```python
from build123d import *

# Parameters (mm, degrees)
SKETCH1_W           = 20
SKETCH1_H           = 20
BOSS_EXTRUDE1_DEPTH = 20
SKETCH2_W           = 10
SKETCH2_H           = 10
CUT_EXTRUDE1_DEPTH  = 20
CUT_EXTRUDE2_DEPTH  = 20


with BuildPart() as part:
    # Sketch1 → Boss-Extrude1 (new body)
    with BuildSketch(Plane.XY):
        with Locations((10, 10)):
            Rectangle(SKETCH1_W, SKETCH1_H)
    extrude(amount=BOSS_EXTRUDE1_DEPTH)

    # Sketch2 → Cut-Extrude1 (cut)
    with BuildSketch(Plane(origin=(0, 20, 0), x_dir=(1, 0, 0), z_dir=(0, 1, 0))):
        with Locations((5, -15)):
            Rectangle(SKETCH2_W, SKETCH2_H)
    extrude(amount=-CUT_EXTRUDE1_DEPTH, mode=Mode.SUBTRACT)

    # Sketch3 → Cut-Extrude2 (cut)
    with BuildSketch(Plane(origin=(0, 20, 0), x_dir=(1, 0, 0), z_dir=(0, 1, 0))):
        Polygon((0, 0), (10, -10), (0, -10), align=None)
    extrude(amount=-CUT_EXTRUDE2_DEPTH, mode=Mode.SUBTRACT)


solid = part.part
```
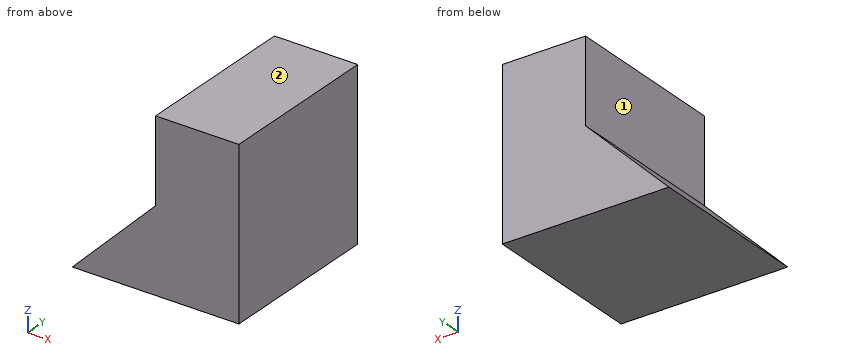
Here's how the part is built. I have some questions about the finished solid (model axes, mm). Face numbers are marked on the shaded views. A direction names the side the tool comes from. Round coordinates to 2 decimals unless told otherwise and drop trailing zeros. Order: outer loops, then holes, each group sorted by start corner. A loop starts at its lowest first (then second) coordinate and runs counter-clockwise, first axis right, second up. Notation, with made-up numbers: M -15.5,-39.5 L -9.5,-39.5 A14 ccw -9.5,-33.5 Z; hole C -31,-38.75 d7. An arc over 180 degrees is marked long. One line per question, with ' | ' between items.
1) I want a section at A-A, the plane z = 8.25. Write out the boundary of the cut face in (x, y).
Working result:
outline: M 8.25,0 L 20,0 L 20,20 L 8.25,20 Z
2) I need wall thicknesses on line 1 along X through (y, z) = (9.5, 12); line 2 along X through (y, z) = (1.5, 8); line 3 along Z through (x, y) = (6.75, 13). Which ranges of each line are inside material? Lowest first, please.
Working result:
line 1: 10 to 20 | line 2: 8 to 20 | line 3: 0 to 6.75
3) For the marked faces 1 and 2, which set-ups out of +Z, -Z, +X, -X, +Y, -Y let a thin tool reach every point of the face, with its end or its side?
Working result:
face 1: +Z, -X, +Y, -Y | face 2: +Z, +X, -X, +Y, -Y
4) I want a section at C-C, the plane x = 1.75. Write out the boundary of the cut face in (y, z), then the cut area to 3 significant figures.
Working result:
outline: M 0,0 L 20,0 L 20,1.75 L 0,1.75 Z | area: 35.0 mm²
5) I want a section at B-B, the plane y = 2. Write out the boundary of the cut face in (x, z), then the cut area to 3 significant figures.
Working result:
outline: M 0,0 L 20,0 L 20,20 L 10,20 L 10,10 Z | area: 250 mm²
6) For pin 1 Ø11 at (y, z) = (10, 15) entering from -X; pin 2 Ø5 at (x, z) = (3.5, 9.5) entering from -Y, each with a flat end and sliding along its axis, tell me the tip position at first contact or that it passes through.
Working result:
pin 1: x = 9.5 | pin 2: through
